The model under review builds one solid part; all positions refer to its coordinate system, in mm. A direction names the side the tool comes from. Round coordinates to 2 decimals unless told otherwise and drop trailing zeros. Write each loop counter-clockwise with the first axis right and the second up, starting at its lowest first coordinate (ties: lowest second). Pieces come first, ordered by that corner, then holes. Notation, with made-up numbers: (55, 50) -> (81, 50) arc R25 cw to (81, 88) -> close; hole circle Ø8 at (73.25, -35.5). An arc over 180 degrees is marked (long way). Return JSON: item names as keys, results as strings. Group by question number.
1. Take a section at D-D, the plane x = -10. Write out the cut boundary in (y, z).
2. For line 1 along Y through (x, z) = (2, 6); line 2 along X through (y, z) = (-10, 4.5); line 3 along Y through (x, z) = (0.5, 4.25), list the stretches that pass through material, from the lowest coordinate up. Write a range as from..to.
3. Take a section at A-A, the plane x = -3. Write out the cut boundary in (y, z), then the cut area to 3 significant figures.
4. Take a section at B-B, the plane y = -3. Write out the cut boundary in (x, z).
5. Tool access review of faces 4 (the cylindrical face through (-16.455, -3.785, 3.451)), 5 (the cylindrical face through (2.301, -17.852, 3.451)): name each direction out of +Z, -Z, +X, -X, +Y, -Y from which nothing blocks a thin tool from reaching the whole face with its end or side.
6. Clearance check with flat-ended pins moving along their axes: P1, Ø4, axis at x = 5, z = 1, coming from the +Y side; P2, Ø1.5, axis at y = 7.5, z = 4.5, coming from the +X side. State where each tip first meets the part, or that it passes through.
7. Mouldability with a two-part tool opening along X and no side actions: class faces 1 (the flat face through (-8, -8, 7)), 2 (the cylindrical face through (14.987, 3.25, 3.451)), 3 (the cylindrical face through (14.31, 10.92, 3.45)) as pulls with the +X half, pulls with the -X half, needs draft (parallel to the pull), parting line crosses it, or undercut.
from build123d import *

# Parameters (mm, degrees)
F0_R     = 11.025
F1_DEPTH = 7


with BuildPart() as f1:
    # F0 (on Top) → F1 (new body)
    with BuildSketch(Plane.XY):
        with BuildLine():
            ThreePointArc((13.820918, -2.232092), (13.955158, -1.119632), (14, 0))
            ThreePointArc((14, 0), (12.124356, 7), (7, 12.124356))
            ThreePointArc((7, 12.124356), (1.119632, 13.955158), (-4.977411, 13.085312))
            ThreePointArc((-4.977411, 13.085312), (-11.525705, 7.947209), (-14, 0))
            ThreePointArc((-14, 0), (-12.645337, -6.007949), (-8.843507, -10.85322))
            ThreePointArc((-8.843507, -10.85322), (-1.119632, -13.955158), (7, -12.124356))
            ThreePointArc((7, -12.124356), (11.525705, -7.947209), (13.820918, -2.232092))
        make_face()
        Circle(F0_R, mode=Mode.SUBTRACT)
        with BuildLine():
            ThreePointArc((-8.843507, -10.85322), (-12.645337, -6.007949), (-14, 0))
            ThreePointArc((-14, 0), (-10.202934, 11.491171), (0, 18))
            ThreePointArc((0, 18), (-9.712436, 15.154821), (-16.35447, 7.518732))
            ThreePointArc((-16.35447, 7.518732), (-16.614557, 6.925063), (-16.853102, 6.322416))
            ThreePointArc((-16.853102, 6.322416), (-16.393457, -3.91863), (-8.843507, -10.85322))
        make_face()
        with BuildLine():
            ThreePointArc((-4.977411, 13.085312), (1.119632, 13.955158), (7, 12.124356))
            ThreePointArc((7, 12.124356), (15.053113, 3.090415), (15.588457, -9))
            ThreePointArc((15.588457, -9), (17.980678, 0.833806), (14.688647, 10.40402))
            ThreePointArc((14.688647, 10.40402), (14.304559, 10.926097), (13.901924, 11.434007))
            ThreePointArc((13.901924, 11.434007), (4.803096, 16.156465), (-4.977411, 13.085312))
        make_face()
        with BuildLine():
            ThreePointArc((2.951178, -17.756423), (11.590361, -12.237835), (13.820918, -2.232092))
            ThreePointArc((13.820918, -2.232092), (11.525705, -7.947209), (7, -12.124356))
            ThreePointArc((7, -12.124356), (-4.850179, -14.581586), (-15.588457, -9))
            ThreePointArc((-15.588457, -9), (-8.268242, -15.988627), (1.665822, -17.922752))
            ThreePointArc((1.665822, -17.922752), (2.309998, -17.85116), (2.951178, -17.756423))
        make_face()
    extrude(amount=F1_DEPTH)


solid = f1.part
Output:
{
 "1": {"outline": "(-14.97, 0) -> (-13.06, 0) -> (-13.06, 7) -> (-14.97, 7) -> close; (-10.37, 0) -> (-4.64, 0) -> (-4.64, 7) -> (-10.37, 7) -> close; (4.64, 0) -> (9.8, 0) -> (9.8, 7) -> (4.64, 7) -> close; (11.75, 0) -> (14.97, 0) -> (14.97, 7) -> (11.75, 7) -> close"},
 "2": {"line 1": "y = -17.89..-14.21, -13.86..-10.84, 10.84..16.11", "line 2": "x = -14.97..-14.58, -10.71..-4.64, 4.64..12.86", "line 3": "y = -17.99..-14.52, -13.99..-11.01, 11.01..15.84"},
 "3": {"outline": "(-17.75, 0) -> (-14.74, 0) -> (-14.74, 7) -> (-17.75, 7) -> close; (-13.67, 0) -> (-10.61, 0) -> (-10.61, 7) -> (-13.67, 7) -> close; (10.61, 0) -> (14.46, 0) -> (14.46, 7) -> (10.61, 7) -> close; (17.03, 0) -> (17.75, 0) -> (17.75, 7) -> (17.03, 7) -> close", "area": "74.5 mm^2"},
 "4": {"outline": "(-16.78, 0) -> (-10.61, 0) -> (-10.61, 7) -> (-16.78, 7) -> close; (10.61, 0) -> (13.93, 0) -> (13.93, 7) -> (10.61, 7) -> close; (16.37, 0) -> (17.75, 0) -> (17.75, 7) -> (16.37, 7) -> close"},
 "5": {"face 4": "+Z, -Z", "face 5": "+Z, -Z, +X, -Y"},
 "6": {"P1": "stops at y = 16.21", "P2": "stops at x = 16.69"},
 "7": {"face 1": "needs draft", "face 2": "undercut", "face 3": "pulls with the +X half"}
}
